from build123d import *

# Parameters (mm, degrees)
SKETCH2_W           = 18.1
SKETCH2_H           = 18.1
SKETCH2_R           = 3
BOSS_EXTRUDE1_DEPTH = 3.75
CUT_EXTRUDE1_START  = 3.75
SKETCH2_3_R         = 7.55
CUT_EXTRUDE1_DEPTH  = 2
SKETCH3_W           = 18.1
SKETCH3_H           = 7.5525
SKETCH3_R           = 1.5
BOSS_EXTRUDE2_DEPTH = 2
BOSS_EXTRUDE3_DEPTH = 1


with BuildPart() as part:
    # Sketch2 → Boss-Extrude1 (new body)
    with BuildSketch(Plane(origin=(0, 0, 0), x_dir=(1, 0, 0), z_dir=(0, 1, 0))):
        with Locations((0, 9.05)):
            Rectangle(SKETCH2_W, SKETCH2_H)
        with Locations(Location((0, 9.05, 0), (0, 0, 270))):
            Circle(SKETCH2_R, mode=Mode.SUBTRACT)
    extrude(amount=BOSS_EXTRUDE1_DEPTH)

    # Sketch2<3> → Cut-Extrude1 (cut)
    with BuildSketch(Plane(origin=(0, 0, 0), x_dir=(1, 0, 0), z_dir=(0, 1, 0)).offset(CUT_EXTRUDE1_START)):
        with Locations(Location((0, 9.05, 0), (0, 0, 270))):
            Circle(SKETCH2_3_R)
    extrude(amount=-CUT_EXTRUDE1_DEPTH, mode=Mode.SUBTRACT)

    # Sketch3 → Boss-Extrude2 (add)
    with BuildSketch(Plane.XY):
        with Locations((0, -3.77625)):
            Rectangle(SKETCH3_W, SKETCH3_H)
        with Locations((4.7625, -3.5525)):
            Circle(SKETCH3_R, mode=Mode.SUBTRACT)
        with Locations((-4.7625, -3.5525)):
            Circle(SKETCH3_R, mode=Mode.SUBTRACT)
    extrude(amount=-BOSS_EXTRUDE2_DEPTH)

    # Sketch5 → Boss-Extrude3 (add, symmetric)
    with BuildSketch(Plane(origin=(0, 0, 0), x_dir=(0, 0, -1), z_dir=(1, 0, 0))):
        with BuildLine():
            Line((2, 0), (2, -7.5525))
            ThreePointArc((2, -7.5525), (3.076392083, -3.267562537), (6.05, 0))
            Line((6.05, 0), (2, 0))
        make_face()
    extrude(amount=BOSS_EXTRUDE3_DEPTH, both=True)


solid = part.part
Design review of the part built by this model. Coordinates are the model's own, in mm. A direction names the side the tool comes from. Round coordinates to 2 decimals unless told otherwise and drop trailing zeros. Order: outer loops, then holes, each group sorted by start corner. A loop starts at its lowest first (then second) coordinate and runs counter-clockwise, first axis right, second up. Notation, with made-up numbers: M 47,89.25 L 103,89.25 A12 ccw 103,108.25 Z; hole C 56,1 d2. An arc over 180 degrees is marked long. Answer as CSV lines item,"result". Start each with the question number.
1) Add section C-C (y = 2.5). Give the boundary of the cut face in (x, z).
2) Add section A-A (z = -9.05). Give the boundary of the cut face in (x, y).
3) The part is to be moulded in two halves that separate along Y. For faces 5 (the face through (-6.26, -3.49, -0.99)), 6 (the face through (0.9, 0.86, -6.19)), 7 (the face through (0, -7.552, -1)), say which applies: +Y half, -Y half, draft (parallel to the pull), parting line (faces both ways), or undercut.
4) Add section B-B (x = -3.5). Give the boundary of the cut face in (y, z), then the cut area to 3 significant figures.
5) For pin 1 Ø4 at (x, y) = (-5.5, -5.5) entering from -Z; pin 2 Ø2 at (y, z) = (-4, -3.5) entering from +X; pin 3 Ø2 at (x, z) = (4.5, -8.5) entering from +Y, all flat-tipped, find the tip position at first contact; note any pin that passes through.
6) Add section D-D (z = -4.5). Give the boundary of the cut face in (x, y).
7) Wall thickness on line 1 along X through (y, z) = (2.2, -9.05); line 2 along X through (y, z) = (0.5, -9.05); line 3 along Y through (x, z) = (7.5, -3.25): over which ranges is each line inside the solid? List them lowest first. Write a range as [from, to].
8) Tool access review of faces 1 (the face through (8, 3.75, -9)), 2 (the face through (-3.2, 1.75, -9.2)), 3 (the face through (5, -5.4, -2)), 4 (the face through (-6, -5, -2)): name each direction out of +Z, -Z, +X, -X, +Y, -Y from which nothing blocks a thin tool from reaching the whole face with its end or side.
Resolved:
1,outline,"M -9.05,-18.1 L 9.05,-18.1 L 9.05,0 L -9.05,0 Z; hole C 0,-9.05 d15.1"
2,outline,"M -9.05,0 L -3,0 L -3,1.75 L -7.55,1.75 L -7.55,3.75 L -9.05,3.75 Z; M 3,0 L 9.05,0 L 9.05,3.75 L 7.55,3.75 L 7.55,1.75 L 3,1.75 Z"
3,face 5,"undercut"
3,face 6,"draft"
3,face 7,"-Y half"
4,outline,"M -7.55,-2 L -4.36,-2 L -4.36,0 L -7.55,0 Z; M -2.74,-2 L 0,-2 L 0,-18.1 L 3.75,-18.1 L 3.75,-15.74 L 1.75,-15.74 L 1.75,-2.36 L 3.75,-2.36 L 3.75,0 L -2.74,0 Z"
4,area,"53.0 mm^2"
5,pin 1,"z = -2"
5,pin 2,"x = 1"
5,pin 3,"y = 1.75"
6,outline,"M -9.05,0 L -1,0 L -1,-1.3 L 1,-1.3 L 1,0 L 9.05,0 L 9.05,3.75 L 6.02,3.75 L 6.02,1.75 L -6.02,1.75 L -6.02,3.75 L -9.05,3.75 Z"
7,line 1,"[-9.05, -7.55], [7.55, 9.05]"
7,line 2,"[-9.05, -3], [3, 9.05]"
7,line 3,"[0, 3.75]"
8,face 1,"+Z, -Z, +X, -X, +Y"
8,face 2,"+Y"
8,face 3,"-Z, +X, -Y"
8,face 4,"-Z, -X, -Y"
